The listing builds one solid part. Answer for the finished solid, in the listing's coordinates (mm). A direction names the side the tool comes from. Coordinates: 2 decimals unless noted, no trailing zeros. Order: outer loops, then holes, each group sorted by start corner. A loop starts at its lowest first (then second) coordinate and runs counter-clockwise, first axis right, second up. Notation, with made-up numbers: (11, -33) -> (67, -33) arc R21 ccw to (67, -22) -> close; hole circle Ø2 at (-34.75, 3.5). An arc over 180 degrees is marked (long way). Return JSON: item names as keys, results as strings.
```python
from build123d import *

# Parameters (mm, degrees)
F0_R     = 17.5
F1_DEPTH = 2
F2_DEPTH = 15
F0_R_2   = 15.5
F3_DEPTH = 10
F4_R     = 5


with BuildPart() as f1:
    # F0 (on Top) → F1 (new body)
    with BuildSketch(Plane.XY):
        with BuildLine():
            Line((34.641016, 25), (-34.641016, 25))
            ThreePointArc((-34.641016, 25), (-38.971143, 22.5), (-38.971143, 17.5))
            Line((-38.971143, 17.5), (-4.330127, -42.5))
            ThreePointArc((-4.330127, -42.5), (0, -45), (4.330127, -42.5))
            Line((4.330127, -42.5), (38.971143, 17.5))
            ThreePointArc((38.971143, 17.5), (38.971143, 22.5), (34.641016, 25))
        make_face()
        with BuildLine():
            ThreePointArc((2, -38), (0, -40), (-2, -38))
            Line((-2, -38), (-2, -30))
            ThreePointArc((-2, -30), (0, -28), (2, -30))
            Line((2, -30), (2, -38))
        make_face(mode=Mode.SUBTRACT)
        with BuildLine():
            ThreePointArc((-33.908965, 17.267949), (-34.641016, 20), (-31.908965, 20.732051))
            Line((-31.908965, 20.732051), (-24.980762, 16.732051))
            ThreePointArc((-24.980762, 16.732051), (-24.248711, 14), (-26.980762, 13.267949))
            Line((-26.980762, 13.267949), (-33.908965, 17.267949))
        make_face(mode=Mode.SUBTRACT)
        with BuildLine():
            Line((-19.052559, 11), (-17.320508, 10))
            ThreePointArc((-17.320508, 10), (0, -20), (17.320508, 10))
            Line((17.320508, 10), (19.052559, 11))
            ThreePointArc((19.052559, 11), (0, -22), (-19.052559, 11))
        make_face(mode=Mode.SUBTRACT)
        Circle(F0_R, mode=Mode.SUBTRACT)
        with BuildLine():
            ThreePointArc((31.908965, 20.732051), (34.641016, 20), (33.908965, 17.267949))
            Line((33.908965, 17.267949), (26.980762, 13.267949))
            ThreePointArc((26.980762, 13.267949), (24.248711, 14), (24.980762, 16.732051))
            Line((24.980762, 16.732051), (31.908965, 20.732051))
        make_face(mode=Mode.SUBTRACT)
    extrude(amount=F1_DEPTH)

    # F0 (on Top) → F2 (join)
    with BuildSketch(Plane.XY):
        with BuildLine():
            ThreePointArc((17.320508, 10), (0, -20), (-17.320508, 10))
            Line((-17.320508, 10), (-19.052559, 11))
            ThreePointArc((-19.052559, 11), (0, -22), (19.052559, 11))
            Line((19.052559, 11), (17.320508, 10))
        make_face()
    extrude(amount=F2_DEPTH)

    # F0 (on Top) → F3 (join)
    with BuildSketch(Plane.XY):
        Circle(F0_R)
        Circle(F0_R_2, mode=Mode.SUBTRACT)
    extrude(amount=F3_DEPTH)

    # F4
    f4_edges = [f1.edges().sort_by_distance(p)[0] for p in [
        (-18.186533, 10.5, 15),
        (18.186533, 10.5, 15),
    ]]
    fillet(f4_edges, radius=F4_R)


solid = f1.part
```
Item 1: The part is cut by section C-C on y = 4. Determine the outline of the cut face in (x, z).
Answer list:
{"outline": "(-31.18, 0) -> (-14.97, 0) -> (-14.97, 10) -> (-17.04, 10) -> (-17.04, 2) -> (-19.6, 2) -> (-19.6, 15) -> (-21.63, 15) -> (-21.63, 2) -> (-31.18, 2) -> close; (14.97, 0) -> (31.18, 0) -> (31.18, 2) -> (21.63, 2) -> (21.63, 15) -> (19.6, 15) -> (19.6, 2) -> (17.04, 2) -> (17.04, 10) -> (14.97, 10) -> close"}
Item 2: The part is cut by section D-D on x = 28.5. Determine the outline of the cut face in (y, z).
Answer list:
{"outline": "(-0.64, 0) -> (14.15, 0) -> (14.15, 2) -> (-0.64, 2) -> close; (18.76, 0) -> (25, 0) -> (25, 2) -> (18.76, 2) -> close"}
Item 3: Which of the six approach directions +Z, -Z, +X, -X, +Y, -Y give full straight-line access (tool end or side, diameter ignored) to faces 5 (the flat face through (-18.17, 10.49, 5.94)), 6 (the cylindrical face through (0.59, -19.99, 8.41)), 7 (the cylindrical face through (0, -28, 1))?
Answer list:
{"face 5": "+Z, +Y", "face 6": "+Z", "face 7": "+Z, -Z"}
Item 4: Flat-ended cylindrical pins translate along their axes: pin 1 (1.6 mm diameter, centred on y = -35.5, z = 0.5, fed in from -X); pin 2 (1.5 mm diameter, centred on x = -8.5, z = 9, fed in from +Y); pin 3 (8 mm diameter, centred on y = 2.5, z = 1.5, fed in from +X). Find the tip coordinate at first contact, or state that the pin passes through.
Answer list:
{"pin 1": "x = -8.83", "pin 2": "y = 15.69", "pin 3": "x = 32.62"}
Item 5: The part is cut by section A-A on z = 4. Determine the outline of the cut face in (x, y).
Answer list:
{"outline": "(-19.05, 11) arc R22 ccw (long way) to (19.05, 11) -> (17.32, 10) arc R20 cw (long way) to (-17.32, 10) -> close; circle Ø35 at (0, 0); hole circle Ø31 at (0, 0)"}
Item 6: The part is cut by section B-B on x = 0. Determine the outline of the cut face in (y, z), plus the area to 3 significant figures.
Answer list:
{"outline": "(-45, 0) -> (-40, 0) -> (-40, 2) -> (-45, 2) -> close; (-28, 0) -> (-15.5, 0) -> (-15.5, 10) -> (-17.5, 10) -> (-17.5, 2) -> (-20, 2) -> (-20, 15) -> (-22, 15) -> (-22, 2) -> (-28, 2) -> close; (15.5, 0) -> (25, 0) -> (25, 2) -> (17.5, 2) -> (17.5, 10) -> (15.5, 10) -> close", "area": "112 mm2"}
Item 7: Determine the mould class of faces 1 (the flat face through (-0.1, -20.4, 15)), 2 (the cylindrical face through (34.619, 20.038, 0.986)), 3 (the cylindrical face through (0, -40, 1)), 4 (the cylindrical face through (-38.934, 22.563, 0.986)) for opening direction Y: pulls with the +Y half, pulls with the -Y half, needs draft (parallel to the pull), parting line crosses it, or undercut.
Answer list:
{"face 1": "needs draft", "face 2": "undercut", "face 3": "undercut", "face 4": "parting line crosses it"}
Item 8: Find the intervals of material crossed by probe 1 along Y at (x, z) = (0, 5); probe 2 along Y at (x, z) = (12, 4.5); probe 3 along X at (y, z) = (-3, 9.75), in increasing order.
Answer list:
{"probe 1": "-22 to -20, -17.5 to -15.5, 15.5 to 17.5", "probe 2": "-18.44 to -16, -12.74 to -9.81, 9.81 to 12.74", "probe 3": "-21.79 to -19.77, -17.24 to -15.21, 15.21 to 17.24, 19.77 to 21.79"}
